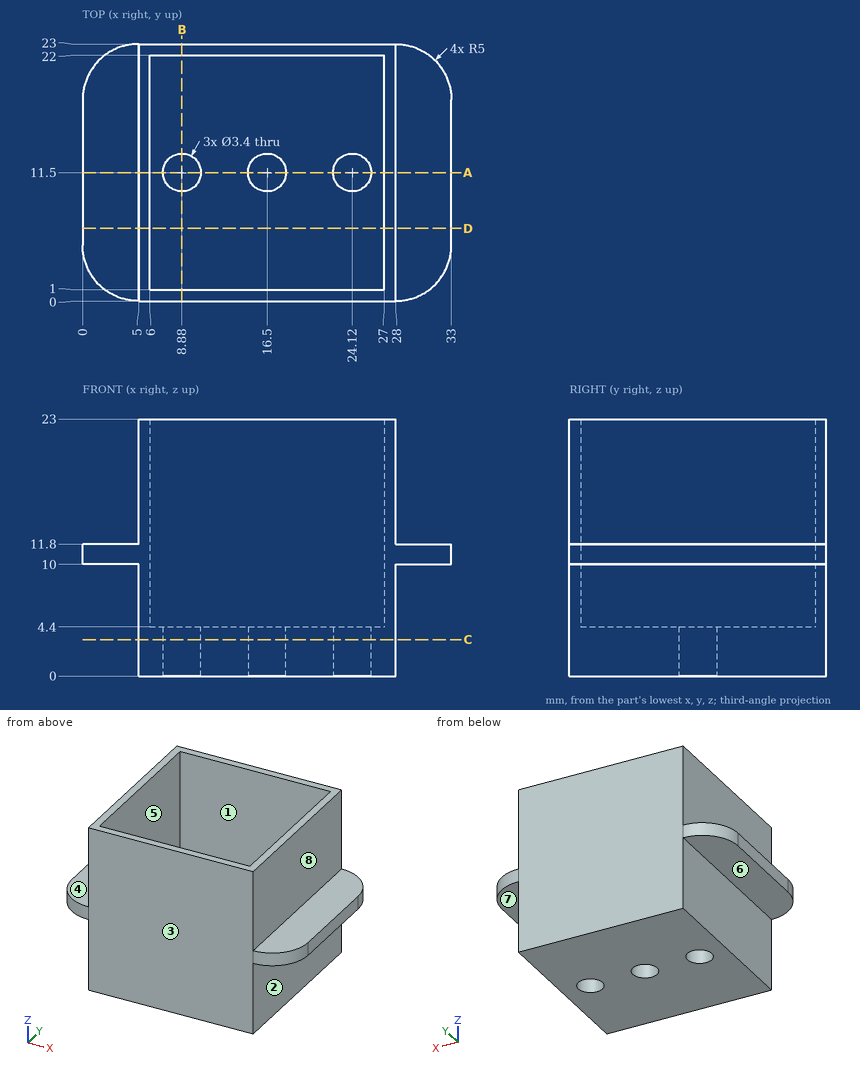
Verification items for this drawing (mm, ordinates from the low corner). A direction names the side the tool comes from. Give positions to 0.01 mm unless a question says otherwise; leave off trailing zeros. Write each loop counter-clockwise with the first axis right and the second up, starting at its lowest first coordinate (ties: lowest second). Pieces come first, ordered by that corner, then holes. Notation, with made-up numbers: (79, 42.25) -> (131, 42.25) arc R21 cw to (131, 54.25) -> close; hole circle Ø10 at (-34, 55.5). An arc over 180 degrees is marked (long way). Use one line per item in the form item = value.
Item 1: Sectioned sample at A-A on y = 11.5. Enter the section's corners in (x, z).
Results list:
outline = (0, 10) -> (5, 10) -> (5, 0) -> (7.18, 0) -> (7.18, 4.4) -> (6, 4.4) -> (6, 23) -> (5, 23) -> (5, 11.8) -> (0, 11.8) -> close; (10.58, 0) -> (14.8, 0) -> (14.8, 4.4) -> (10.58, 4.4) -> close; (18.2, 0) -> (22.42, 0) -> (22.42, 4.4) -> (18.2, 4.4) -> close; (25.82, 0) -> (28, 0) -> (28, 10) -> (33, 10) -> (33, 11.8) -> (28, 11.8) -> (28, 23) -> (27, 23) -> (27, 4.4) -> (25.82, 4.4) -> close
Item 2: Depth check by flat-ended pin: pin 1 Ø1.5 at (x, y) = (30, 17) entering from +Z; pin 2 Ø2.5 at (x, y) = (24.12, 11.5) entering from +Z; pin 3 Ø3 at (y, z) = (15, 16) entering from +X; pin 4 Ø3 at (y, z) = (11, 6.5) entering from -X. Enter the tip coordinate at first touch or a pass-through.
Results list:
pin_1 = 11.8
pin_2 = through
pin_3 = 28
pin_4 = 5
Item 3: Mould release check, pull along Y, two halves, no side actions. Record for the marked faces 1, 2 and 3: released by +Y, released by -Y, zero draft, split by the parting line, or undercut.
Results list:
face_1 = undercut
face_2 = zero draft
face_3 = released by -Y
Item 4: Sectioned sample at C-C on z = 3.25. Enter the section's corners in (x, y), plus the area to 3 significant figures.
Results list:
outline = (5, 0) -> (28, 0) -> (28, 23) -> (5, 23) -> close; hole circle Ø3.4 at (8.88, 11.5); hole circle Ø3.4 at (16.5, 11.5); hole circle Ø3.4 at (24.12, 11.5)
area = 502 mm2
Item 5: Sectioned sample at B-B on x = 8.88. Enter the section's corners in (y, z), plus the area to 3 significant figures.
Results list:
outline = (0, 0) -> (9.8, 0) -> (9.8, 4.4) -> (1, 4.4) -> (1, 23) -> (0, 23) -> close; (13.2, 0) -> (23, 0) -> (23, 23) -> (22, 23) -> (22, 4.4) -> (13.2, 4.4) -> close
area = 123 mm2
Item 6: Scan lines: line 1 (X direction, y = 11.5, z = 2.5); line 2 (Y direction, x = 14.5, z = 14.25); line 3 (Y direction, x = 8.88, z = 2). Record each from-to range of solid material in increasing order.
Results list:
line_1 = 5 to 7.18, 10.58 to 14.8, 18.2 to 22.42, 25.82 to 28
line_2 = 0 to 1, 22 to 23
line_3 = 0 to 9.8, 13.2 to 23
Item 7: Access from +Z, -Z, +X, -X, +Y, -Y to the whole of each face (thin tool, end or side, straight path). Record for the marked faces 4, 5, 6, 7 and 8.
Results list:
face_4 = +Z, -X, +Y, -Y
face_5 = +Z
face_6 = -Z, -X, +Y, -Y
face_7 = -Z, +X, +Y, -Y
face_8 = +Z, +X, +Y, -Y
Item 8: Sectioned sample at D-D on y = 6.5. Enter the section's corners in (x, z), plus the area to 3 significant figures.
Results list:
outline = (0, 10) -> (5, 10) -> (5, 0) -> (28, 0) -> (28, 10) -> (33, 10) -> (33, 11.8) -> (28, 11.8) -> (28, 23) -> (27, 23) -> (27, 4.4) -> (6, 4.4) -> (6, 23) -> (5, 23) -> (5, 11.8) -> (0, 11.8) -> close
area = 156 mm2
